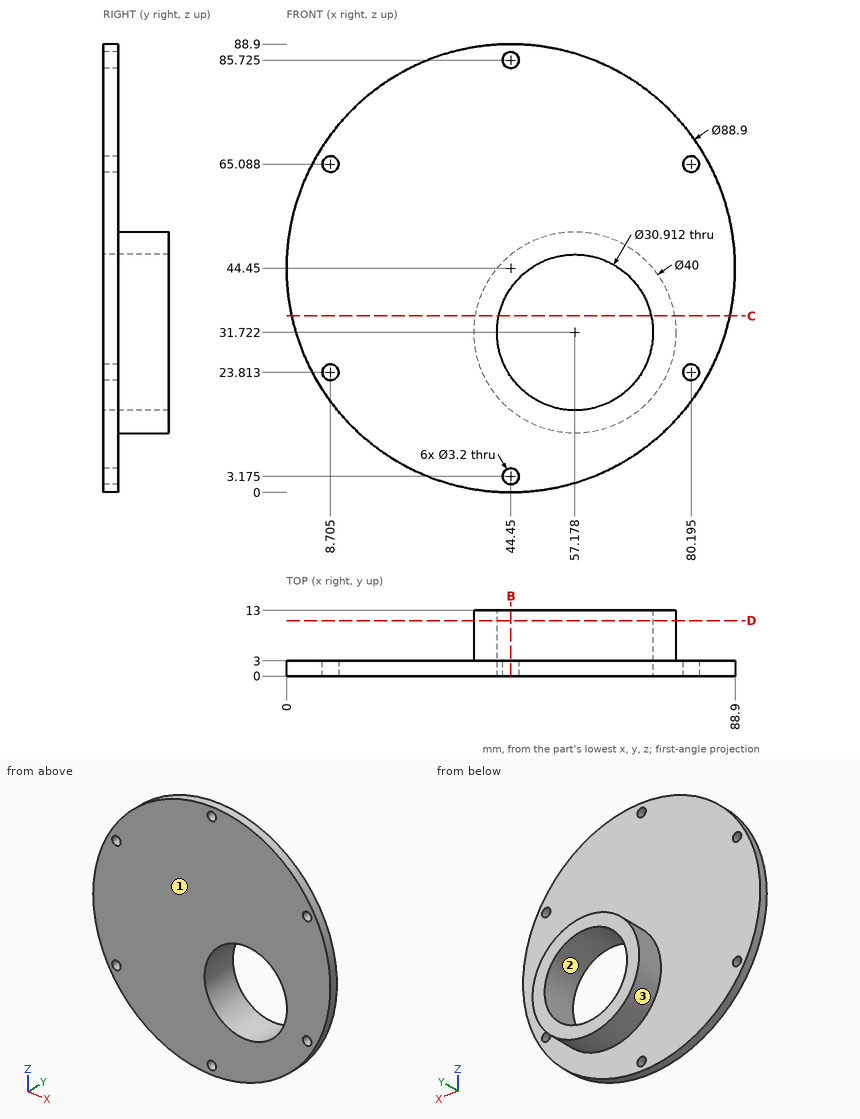
Geometry check sheet. Reference: drawing and pictorial views, mm from the part's lowest x, y, z. Round coordinates to 2 decimals unless told otherwise and drop trailing zeros. Loops run counter-clockwise (first coordinate to the right, second up) from the corner with the lowest first, then second, coordinate; pieces in that order, holes last. Notation, with made-up numbers: (-31.75, 80.5) - (5.25, 80.5) arc R29 ccw to (5.25, 101.5) - close; hole circle Ø9 at (2.25, 79). An arc over 180 degrees is marked (long way). Use a Markdown table: item, result. Add a question column.
1. Release check for a two-part mould opening along Z. For the marked faces 1, 2 and 3 record: released by +Z, released by -Z, zero draft, split by the parting line, or undercut.
2. Section check C-C, the plane z = 35. Record the boundary of the cut face in (x, y).
3. Gauge pin test, flat ends, axial feed: pin 1 (5 mm diameter, centred on x = 44, y = 4.5, fed in from +Z); pin 2 (3.5 mm diameter, centred on x = 44.45, z = 85.725, fed in from +Y); pin 3 (5 mm diameter, centred on x = 70, y = 9, fed in from +Z). Record the tip position at first contact, or that the pin passes through.
4. Section check D-D, the plane y = 11. Record the boundary of the cut face in (x, z) (1 decimal), plus the area to 3 significant figures.
5. Section check B-B, the plane x = 44.45. Give the number of separate pieces and of enclosed holes in the cut face, plus the area to 3 significant figures.
6. Thickness scan on probe 1 along X at (y, z) = (2.5, 65.5); probe 2 along X at (y, z) = (1.75, 23.5) (1 decimal); probe 3 along Y at (x, z) = (85, 55). Record the ranges inside material, lowest first. Write a range as [from, to].
Checks:
| question | item | result |
|---|---|---|
| 1 | face 1 | zero draft |
| 1 | face 2 | undercut |
| 1 | face 3 | split by the parting line |
| 2 | outline | (1.02, 0) - (42.07, 0) - (42.07, 13) - (37.45, 13) - (37.45, 3) - (1.02, 3) - close; (72.28, 0) - (87.88, 0) - (87.88, 3) - (76.91, 3) - (76.91, 13) - (72.28, 13) - close |
| 3 | pin 1 | stops at z = 88.9 |
| 3 | pin 2 | stops at y = 3 |
| 3 | pin 3 | stops at z = 48.85 |
| 4 | outline | circle Ø40 at (57.2, 31.7); hole circle Ø30.9 at (57.2, 31.7) |
| 4 | area | 506 mm^2 |
| 5 | separate pieces | 4 |
| 5 | enclosed holes | 0 |
| 5 | area | 328 mm^2 |
| 6 | probe 1 | x = [5.3, 7.16], [10.25, 78.65], [81.74, 83.6] |
| 6 | probe 2 | x = [5.2, 7.1], [10.3, 44.1], [70.3, 78.6], [81.8, 83.7] |
| 6 | probe 3 | y = [0, 3] |
